Design review of the part built by this model. Coordinates are the model's own, in mm. A direction names the side the tool comes from. Give positions to 0.01 mm unless a question says otherwise; leave off trailing zeros. Order: outer loops, then holes, each group sorted by start corner. A loop starts at its lowest first (then second) coordinate and runs counter-clockwise, first axis right, second up. Notation, with made-up numbers: (-22.75, 9.5) -> (-7.75, 9.5) arc R18 cw to (-7.75, 29.5) -> close; hole circle Ø2 at (89.25, 48.25). An arc over 180 degrees is marked (long way). Answer in a Markdown table with one row per item. Add a question column.
```python
from build123d import *

# Parameters (mm, degrees)
AUFSATZ_LINEAR_AUSTRAGEN1_DEPTH  = 18.05
SKIZZE3_R                        = 4.14
SCHNITT_LINEAR_AUSTRAGEN1_DEPTH  = 12.725
SKIZZE4_R                        = 4.14
SCHNITT_LINEAR_AUSTRAGEN2_DEPTH  = 2
AUFSATZ_LINEAR_AUSTRAGEN2_DEPTH  = 1
LINEARES_MUSTER6_COUNT           = 3
LINEARES_MUSTER6_PITCH           = 35
LINEARES_MUSTER6_COPY_1_SKETCH_R = 4.14
LINEARES_MUSTER6_COPY_1_DEPTH    = 2
LINEARES_MUSTER6_COPY_2_SKETCH_R = 4.14
LINEARES_MUSTER6_COPY_2_DEPTH    = 2


with BuildPart() as part:
    # Skizze1 → Aufsatz-Linear austragen1 (new, symmetric)
    with BuildSketch(Plane.XY):
        with BuildLine():
            ThreePointArc((-8.350956521, 9.600907291), (-23.24, 0), (-8.350956521, -9.600907291))
            ThreePointArc((-8.350956521, -9.600907291), (0, -7.797678049), (8.350956521, -9.600907291))
            ThreePointArc((8.350956521, -9.600907291), (23.24, 0), (8.350956521, 9.600907291))
            ThreePointArc((8.350956521, 9.600907291), (0, 7.797678049), (-8.350956521, 9.600907291))
        make_face()
    aufsatz_linear_austragen1 = extrude(amount=AUFSATZ_LINEAR_AUSTRAGEN1_DEPTH, both=True)

    # Skizze3 → Schnitt-Linear austragen1 (cut, symmetric)
    with BuildSketch(Plane.XY):
        with BuildLine():
            ThreePointArc((-8.350956521, 9.600907291), (-23.24, 0), (-8.350956521, -9.600907291))
            ThreePointArc((-8.350956521, -9.600907291), (0, -7.797678049), (8.350956521, -9.600907291))
            ThreePointArc((8.350956521, -9.600907291), (23.24, 0), (8.350956521, 9.600907291))
            ThreePointArc((8.350956521, 9.600907291), (0, 7.797678049), (-8.350956521, 9.600907291))
        make_face()
        with Locations((-12.7, 0)):
            Circle(SKIZZE3_R, mode=Mode.SUBTRACT)
        with Locations((12.7, 0)):
            Circle(SKIZZE3_R, mode=Mode.SUBTRACT)
    schnitt_linear_austragen1 = extrude(amount=SCHNITT_LINEAR_AUSTRAGEN1_DEPTH, both=True, mode=Mode.SUBTRACT)

    # Skizze4 → Schnitt-Linear austragen2 (cut)
    with BuildSketch(Plane.XY.offset(18.05)):
        with BuildLine():
            ThreePointArc((-8.350956521, 9.600907291), (-23.24, 0), (-8.350956521, -9.600907291))
            ThreePointArc((-8.350956521, -9.600907291), (0, -7.797678049), (8.350956521, -9.600907291))
            ThreePointArc((8.350956521, -9.600907291), (23.24, 0), (8.350956521, 9.600907291))
            ThreePointArc((8.350956521, 9.600907291), (0, 7.797678049), (-8.350956521, 9.600907291))
        make_face()
        with Locations((-12.7, 0)):
            Circle(SKIZZE4_R, mode=Mode.SUBTRACT)
        with Locations((12.7, 0)):
            Circle(SKIZZE4_R, mode=Mode.SUBTRACT)
    schnitt_linear_austragen2 = extrude(amount=-SCHNITT_LINEAR_AUSTRAGEN2_DEPTH, mode=Mode.SUBTRACT)

    # Spiegeln1: Schnitt-Linear austragen2 across plane
    add(schnitt_linear_austragen2.mirror(Plane.XY), mode=Mode.SUBTRACT)

    # Skizze5 → Aufsatz-Linear austragen2 (add)
    with BuildSketch(Plane.XY.offset(16.05)):
        with BuildLine():
            Line((-18.67281729, 4.583103901), (-15.984482829, 2.520272316))
            ThreePointArc((-15.984482829, 2.520272316), (-14.531075178, 3.71305315), (-12.7, 4.14))
            Line((-12.7, 4.14), (-8.56, 4.14))
            Line((-8.56, 4.14), (-7.120601032, 5.528571429))
            Line((-7.120601032, 5.528571429), (7.120601032, 5.528571429))
            Line((7.120601032, 5.528571429), (8.56, 4.14))
            Line((8.56, 4.14), (12.7, 4.14))
            ThreePointArc((12.7, 4.14), (16.84, 0), (12.7, -4.14))
            Line((12.7, -4.14), (8.56, -4.14))
            Line((8.56, -4.14), (7.120601032, -5.528571429))
            Line((7.120601032, -5.528571429), (-7.120601032, -5.528571429))
            Line((-7.120601032, -5.528571429), (-8.56, -4.14))
            Line((-8.56, -4.14), (-12.7, -4.14))
            ThreePointArc((-12.7, -4.14), (-14.531075178, -3.71305315), (-15.984482829, -2.520272316))
            Line((-15.984482829, -2.520272316), (-18.67281729, -4.583103901))
            ThreePointArc((-18.67281729, -4.583103901), (-16.029801996, -6.752170497), (-12.7, -7.528571429))
            Line((-12.7, -7.528571429), (12.7, -7.528571429))
            ThreePointArc((12.7, -7.528571429), (20.228571429, 0), (12.7, 7.528571429))
            Line((12.7, 7.528571429), (-12.7, 7.528571429))
            ThreePointArc((-12.7, 7.528571429), (-16.029801996, 6.752170497), (-18.67281729, 4.583103901))
        make_face()
    extrude(amount=AUFSATZ_LINEAR_AUSTRAGEN2_DEPTH)

    # Lineares Muster6: Aufsatz-Linear austragen1, Schnitt-Linear austragen1, Schnitt-Linear austragen2 ×3
    with Locations(*[(0, 0, -i * LINEARES_MUSTER6_PITCH) for i in range(1, LINEARES_MUSTER6_COUNT)]):
        add(aufsatz_linear_austragen1)
        add(schnitt_linear_austragen1, mode=Mode.SUBTRACT)
        add(schnitt_linear_austragen2, mode=Mode.SUBTRACT)

    # Lineares Muster6 copy 1 sketch → Lineares Muster6 copy 1 (cut)
    with BuildSketch(Plane(origin=(0, 0, -53.05), x_dir=(1, 0, 0), z_dir=(0, 0, -1))):
        with BuildLine():
            ThreePointArc((-8.350956521, -9.600907291), (-23.24, 0), (-8.350956521, 9.600907291))
            ThreePointArc((-8.350956521, 9.600907291), (0, 7.797678049), (8.350956521, 9.600907291))
            ThreePointArc((8.350956521, 9.600907291), (23.24, 0), (8.350956521, -9.600907291))
            ThreePointArc((8.350956521, -9.600907291), (0, -7.797678049), (-8.350956521, -9.600907291))
        make_face()
        with Locations((-12.7, 0)):
            Circle(LINEARES_MUSTER6_COPY_1_SKETCH_R, mode=Mode.SUBTRACT)
        with Locations((12.7, 0)):
            Circle(LINEARES_MUSTER6_COPY_1_SKETCH_R, mode=Mode.SUBTRACT)
    extrude(amount=-LINEARES_MUSTER6_COPY_1_DEPTH, mode=Mode.SUBTRACT)

    # Lineares Muster6 copy 2 sketch → Lineares Muster6 copy 2 (cut)
    with BuildSketch(Plane(origin=(0, 0, -88.05), x_dir=(1, 0, 0), z_dir=(0, 0, -1))):
        with BuildLine():
            ThreePointArc((-8.350956521, -9.600907291), (-23.24, 0), (-8.350956521, 9.600907291))
            ThreePointArc((-8.350956521, 9.600907291), (0, 7.797678049), (8.350956521, 9.600907291))
            ThreePointArc((8.350956521, 9.600907291), (23.24, 0), (8.350956521, -9.600907291))
            ThreePointArc((8.350956521, -9.600907291), (0, -7.797678049), (-8.350956521, -9.600907291))
        make_face()
        with Locations((-12.7, 0)):
            Circle(LINEARES_MUSTER6_COPY_2_SKETCH_R, mode=Mode.SUBTRACT)
        with Locations((12.7, 0)):
            Circle(LINEARES_MUSTER6_COPY_2_SKETCH_R, mode=Mode.SUBTRACT)
    extrude(amount=-LINEARES_MUSTER6_COPY_2_DEPTH, mode=Mode.SUBTRACT)


solid = part.part
```
1) Machinability: for faces 5 (the face through (0, 0, 16.05)), 6 (the face through (0, 0, -12.725)), 7 (the face through (20.227, -0.166, 16.543)), 8 (the face through (-16.07, -6.73, 16.54)), 9 (the face through (-0.12, -7.8, -84.36)), which of the approach directions +Z, -Z, +X, -X, +Y, -Y give a long, thin tool a straight path to every point of the face, cutting with its end or side? Answer none if there is none.
2) Mouldability with a two-part tool opening along Y and no side actions: class faces 1 (the face through (0, 0, -82.725)), 2 (the face through (8.564, 0.182, 17.286)), 3 (the face through (0.12, 7.8, -84.36)), 4 (the face through (-8.75, 1.24, -0.18)) as +Y half, -Y half, draft (parallel to the pull), parting line (faces both ways), or undercut.
3) Add section B-B, the plane z = -33. Write out the cut boundary in (x, y).
4) Clearance check with flat-ended pins moving along their axes: P1, Ø3, axis at x = 10.5, z = -6, coming from the +Y side; P2, Ø1, axis at y = -5, z = -46.5, coming from the -X side; P3, Ø6.5, axis at x = -3.5, y = -5, coming from the +Z side; P4, Ø1.1, axis at x = 0.5, z = 16.5, coming from the -Y side. State where each tip first meets the part, or that it passes through.
5) For L1, parallel to Z at x = 5, y = 7.25 (3 decimals); L2, parallel to Z at x = -15, y = 9.5 (3 decimals); L3, parallel to X at y = -1.25, z = 9, list the stretches that pass through material, from the lowest coordinate up.
6) Add section A-A, the plane x = 6. Give the number of separate pieces and of enclosed holes in the cut face, and give its area (3 significant figures).
Verdict:
| question | item | result |
|---|---|---|
| 1 | face 5 | +Z |
| 1 | face 6 | none |
| 1 | face 7 | +Z, +X |
| 1 | face 8 | +Z, -X, -Y |
| 1 | face 9 | +Z, -Z, -Y |
| 2 | face 1 | draft |
| 2 | face 2 | undercut |
| 2 | face 3 | +Y half |
| 2 | face 4 | parting line |
| 3 | outline | circle Ø8.28 at (-12.7, 0); circle Ø8.28 at (12.7, 0) |
| 4 | P1 | stops at y = 4.08 |
| 4 | P2 | passes through |
| 4 | P3 | stops at z = 17.05 |
| 4 | P4 | stops at y = -7.81 |
| 5 | L1 | z = -86.05 to -82.725, -57.275 to -53.95, -51.05 to -47.725, -22.275 to -18.95, -16.05 to -12.725, 12.725 to 17.05 |
| 5 | L2 | z = -86.05 to -82.725, -57.275 to -53.95, -51.05 to -47.725, -22.275 to -18.95, -16.05 to -12.725, 12.725 to 16.05 |
| 5 | L3 | x = -16.65 to -8.75, 8.75 to 16.65 |
| 6 | separate pieces | 6 |
| 6 | enclosed holes | 0 |
| 6 | area | 351 mm2 |
